Build history of the part. All positions in model axes, mm. A direction names the side the tool comes from. Give positions to 0.01 mm unless a question says otherwise; leave off trailing zeros. Write each loop counter-clockwise with the first axis right and the second up, starting at its lowest first coordinate (ties: lowest second). Pieces come first, ordered by that corner, then holes.
from build123d import *

# Parameters (mm, degrees)
BOSS_EXTRUDE1_DEPTH   = 15
BOSS_EXTRUDE1_2_DEPTH = 15
SKETCH2_W             = 9
SKETCH2_H             = 25
BOSS_EXTRUDE2_DEPTH   = 3
BOSS_EXTRUDE3_START   = 3
BOSS_EXTRUDE3_DEPTH   = 3
SKETCH4_W             = 3
SKETCH4_H             = 15.397275821
CUT_EXTRUDE1_DEPTH    = 6
BOSS_EXTRUDE4_DEPTH   = 18
SKETCH7_W             = 11
SKETCH7_H             = 3
BOSS_EXTRUDE5_DEPTH   = 12.25
CHAMFER1_SIZE         = 2
SKETCH8_W             = 15
SKETCH8_H             = 5
BOSS_EXTRUDE6_DEPTH   = 10
SKETCH9_R             = 2.0625
CUT_EXTRUDE2_DEPTH    = 52.662365412


with BuildPart() as part:
    # Sketch1 → Boss-Extrude1 (new body)
    with BuildSketch(Plane.XY):
        Polygon((0, 43), (0, 0), (15, 0), (15, -12), (18, -12), (18, 3), (3, 3), (3, 43), align=None)
    extrude(amount=BOSS_EXTRUDE1_DEPTH)



with BuildPart() as body_2:
    # Sketch1 → Boss-Extrude1 2 (new body)
    with BuildSketch(Plane.XY):
        with BuildLine():
            Line((0, -9), (0, -12))
            ThreePointArc((0, -12), (-8.485281374, -8.485281374), (-12, 0))
            Line((-12, 0), (-12, 43))
            Line((-12, 43), (-9, 43))
            Line((-9, 43), (-9, 0))
            ThreePointArc((-9, 0), (-6.363961031, -6.363961031), (0, -9))
        make_face()
    extrude(amount=BOSS_EXTRUDE1_2_DEPTH)


with BuildPart() as part_1:
    add(part.part)

    add(body_2.part)  # Boss-Extrude2 merges body 2
    # Sketch2 → Boss-Extrude2 (add)
    with BuildSketch(Plane(origin=(0, 0, 0), x_dir=(-1, 0, 0), z_dir=(0, 0, -1))):
        with BuildLine():
            Line((-3, 43), (12, 43))
            Line((12, 43), (12, 0))
            ThreePointArc((12, 0), (8.485281374, -8.485281374), (0, -12))
            Line((0, -12), (-18, -12))
            Line((-18, -12), (-18, 3))
            Line((-18, 3), (-3, 3))
            Line((-3, 3), (-3, 43))
        make_face()
        with Locations((4.5, 15.5)):
            Rectangle(SKETCH2_W, SKETCH2_H, mode=Mode.SUBTRACT)
    extrude(amount=BOSS_EXTRUDE2_DEPTH)

    # Sketch3 → Boss-Extrude3 (add)
    with BuildSketch(Plane.XY.offset(15).offset(BOSS_EXTRUDE3_START)):
        with BuildLine():
            Line((-12, 0), (-12, 43))
            Line((-12, 43), (3, 43))
            Line((3, 43), (3, 3))
            Line((3, 3), (18, 3))
            Line((18, 3), (18, -12))
            Line((18, -12), (0, -12))
            ThreePointArc((0, -12), (-8.485281374, -8.485281374), (-12, 0))
        make_face()
    extrude(amount=-BOSS_EXTRUDE3_DEPTH)

    # Sketch4 → Cut-Extrude1 (cut)
    with BuildSketch(Plane(origin=(0, 0, -3), x_dir=(-1, 0, 0), z_dir=(0, 0, -1))):
        with Locations((-1.5, 16.998637911)):
            Rectangle(SKETCH4_W, SKETCH4_H)
    extrude(amount=-CUT_EXTRUDE1_DEPTH, mode=Mode.SUBTRACT)

    # Sketch5 → Boss-Extrude4 (add)
    with BuildSketch(Plane(origin=(3, 0, 0), x_dir=(0, 0, -1), z_dir=(1, 0, 0))):
        Polygon((-3, 32.347275821), (-3, 8.347275821), (-3, 5.347275821), (-7, 5.347275821), (-7, 8.347275821), (-7, 32.347275821), (-7, 35.347275821), (-3, 35.347275821), align=None)
    extrude(amount=BOSS_EXTRUDE4_DEPTH)

    # Sketch7 → Boss-Extrude5 (add)
    with BuildSketch(Plane(origin=(0, 0, 3), x_dir=(-1, 0, 0), z_dir=(0, 0, -1))):
        with Locations((-15.5, 33.847275821)):
            Rectangle(SKETCH7_W, SKETCH7_H)
        with Locations((-15.5, 6.847275821)):
            Rectangle(SKETCH7_W, SKETCH7_H)
    extrude(amount=BOSS_EXTRUDE5_DEPTH)

    # Chamfer1
    chamfer1_edges = [part_1.edges().sort_by_distance(p)[0] for p in [
        (0, 43, 7.5),
        (-4.5, 43, 0),
        (-9, 43, 7.5),
        (-4.5, 43, 15),
    ]]
    chamfer(chamfer1_edges, length=CHAMFER1_SIZE)

    # Sketch8 → Boss-Extrude6 (add)
    with BuildSketch(Plane.XY.offset(18)):
        with Locations((-4.5, 2.5)):
            Rectangle(SKETCH8_W, SKETCH8_H)
    extrude(amount=BOSS_EXTRUDE6_DEPTH)

    # Sketch9 → Cut-Extrude2 (cut, through all)
    with BuildSketch(Plane(origin=(0, 5, 0), x_dir=(1, 0, 0), z_dir=(0, 1, 0))):
        with Locations(Location((-8.25, -23, 0), (0, 0, 270))):
            Circle(SKETCH9_R)
        with Locations(Location((-0.75, -23, 0), (0, 0, 270))):
            Circle(SKETCH9_R)
    extrude(amount=-CUT_EXTRUDE2_DEPTH, mode=Mode.SUBTRACT)


solid = part_1.part
(1) Mould opens along Z. For faces 1 (the face through (-4, 3, -1)), 2 (the face through (-0.66, 2.54, 20.94)), 3 (the face through (-5, 3, 28)) say: +Z half, -Z half, draft (parallel to the pull), parting line (faces both ways), or undercut.
(2) Saw through at C-C, the plane y = 30. List the corners of the cut face in (x, z).
(3) Probe line 1 (X direction, y = 1, z = 23); line 2 (X direction, y = 9, z = 0); line 3 (Z direction, x = -5.5, y = 30). List the from-to ranges inside material, lowest first.
(4) Drop flat-ended pins along their axis: pin 1 (6 mm diameter, centred on y = 11, z = 16, fed in from +X); pin 2 (7.5 mm diameter, centred on x = -2.5, y = 19, fed in from +Z); pin 3 (0.9 mm diameter, centred on y = 7, z = -4, fed in from -X). Give the stop position or say it passes through.
(5) Saw through at B-B, the plane y = 1.5. Give the number of separate pieces and of enclosed holes in the cut face, plus the area to 3 significant figures.
(6) Saw through at D-D, the plane z = 2. List the corners of the cut face in (x, y).
(7) 3-axis set-ups, long thin cutter, end or side, ignore diameter. For faces 4 (the face through (10, 3, 8)), 5 (the face through (7, 0, 7)), 6 (the face through (-5, 35, 0)), 7 (the face through (-4, 28, -1)), 8 (the face through (18, -4, 8)): which of +Z, -Z, +X, -X, +Y, -Y reach the whole face in a straight line?
(8) Saw through at A-A, the plane z = -4.5. List the corners of the cut face in (x, y).
Computed values:
1. face 1: draft
1. face 2: undercut
1. face 3: +Z half
2. outline: (-12, -3) - (3, -3) - (3, 3) - (21, 3) - (21, 7) - (3, 7) - (3, 18) - (-12, 18) - close; hole (-9, 0) - (0, 0) - (0, 15) - (-9, 15) - close
3. line 1: x = -12 to -10.31, -6.19 to -2.81, 1.31 to 3
3. line 2: x = -12 to -9, 0 to 3
3. line 3: z = -3 to 0, 15 to 18
4. pin 1: stops at x = 3
4. pin 2: stops at z = 18
4. pin 3: stops at x = 10
5. separate pieces: 1
5. enclosed holes: 3
5. area: 618 mm2
6. outline: (-12, 0) arc R12 ccw to (0, -12) - (0, -9) arc R9 cw to (-9, 0) - (-9, 41) - (-11, 43) - (-12, 43) - close; (0, 0) - (15, 0) - (15, -12) - (18, -12) - (18, 3) - (3, 3) - (3, 9.3) - (0, 9.3) - close; (0, 24.7) - (3, 24.7) - (3, 43) - (2, 43) - (0, 41) - close; (10, 5.35) - (21, 5.35) - (21, 8.35) - (10, 8.35) - close; (10, 32.35) - (21, 32.35) - (21, 35.35) - (10, 35.35) - close
7. face 4: +Z, -Z, +X
7. face 5: -Y
7. face 6: +Y
7. face 7: -Z
7. face 8: +Z, -Z, +X, -Y
8. outline: (10, 5.35) - (21, 5.35) - (21, 8.35) - (10, 8.35) - close; (10, 32.35) - (21, 32.35) - (21, 35.35) - (10, 35.35) - close
